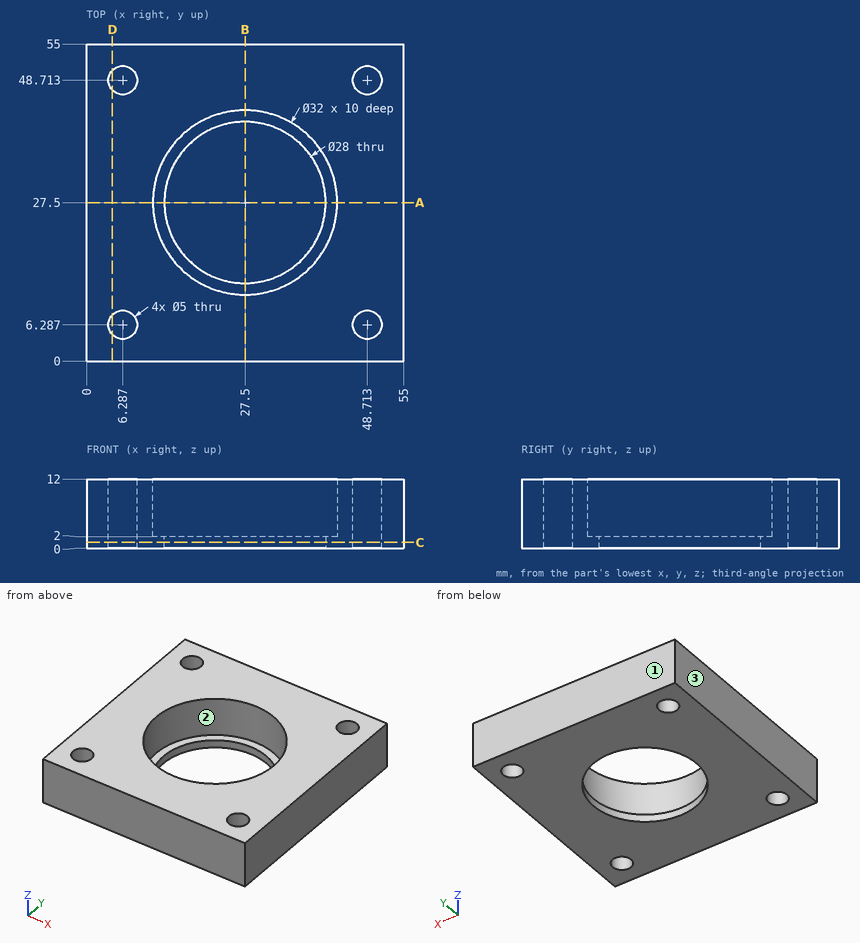
Study the drawing (mm; zero at the part's minimum x, y, z) and answer. Round coordinates to 2 decimals unless told otherwise and drop trailing zeros. Loops run counter-clockwise (first coordinate to the right, second up) from the corner with the lowest first, then second, coordinate; pieces in that order, holes last. Notation, with made-up numbers: (27, 16) -> (77, 16) arc R32 ccw to (77, 43) -> close; hole circle Ø5 at (54, 53). An arc over 180 degrees is marked (long way). Use one line per item in the form item = value.
1. For a pull along X with two mould halves and no side action, classify the marked faces 1, 2 and 3 as released by +X, released by -X, zero draft, split by the parting line, or undercut.
Answer key:
face_1 = zero draft
face_2 = undercut
face_3 = released by -X
2. Find the intervals of material crossed by probe 1 along X at (y, z) = (7.5, 5.5); probe 2 along X at (y, z) = (28, 1); probe 3 along X at (y, z) = (4, 8.75) (1 decimal), in increasing order. Write a range as [from, to].
Answer key:
probe_1 = [0, 4.1], [8.47, 46.53], [50.9, 55]
probe_2 = [0, 13.51], [41.49, 55]
probe_3 = [0, 5.3], [7.3, 47.7], [49.7, 55]
3. The part is cut by section A-A on y = 27.5. Determine the outline of the cut face in (x, z), and give its area (3 significant figures).
Answer key:
outline = (0, 0) -> (13.5, 0) -> (13.5, 2) -> (11.5, 2) -> (11.5, 12) -> (0, 12) -> close; (41.5, 0) -> (55, 0) -> (55, 12) -> (43.5, 12) -> (43.5, 2) -> (41.5, 2) -> close
area = 284 mm²
4. The part is cut by section D-D on x = 4.5. Determine the outline of the cut face in (y, z) (1 decimal), and give its area (3 significant figures).
Answer key:
outline = (0, 0) -> (4.5, 0) -> (4.5, 12) -> (0, 12) -> close; (8, 0) -> (47, 0) -> (47, 12) -> (8, 12) -> close; (50.5, 0) -> (55, 0) -> (55, 12) -> (50.5, 12) -> close
area = 576 mm²
5. The part is cut by section C-C on z = 1. Determine the outline of the cut face in (x, y).
Answer key:
outline = (0, 0) -> (55, 0) -> (55, 55) -> (0, 55) -> close; hole circle Ø5 at (6.29, 6.29); hole circle Ø5 at (6.29, 48.71); hole circle Ø28 at (27.5, 27.5); hole circle Ø5 at (48.71, 6.29); hole circle Ø5 at (48.71, 48.71)
